```python
from build123d import *

# Parameters (mm, degrees)
SKETCH1_W           = 400
SKETCH1_H           = 300
BOSS_EXTRUDE1_DEPTH = 7.62
CUT_EXTRUDE1_DEPTH  = 7.62
CUT_EXTRUDE2_DEPTH  = 7.62


with BuildPart() as part:
    # Sketch1 → Boss-Extrude1 (new body)
    with BuildSketch(Plane(origin=(0, 0, 0), x_dir=(1, 0, 0), z_dir=(0, 1, 0))):
        with Locations((200, 150)):
            Rectangle(SKETCH1_W, SKETCH1_H)
    extrude(amount=BOSS_EXTRUDE1_DEPTH)

    # Sketch2 → Cut-Extrude1 (cut)
    with BuildSketch(Plane(origin=(0, 7.62, 0), x_dir=(1, 0, 0), z_dir=(0, 1, 0))):
        with BuildLine():
            ThreePointArc((32.1719512, 167.526), (25, 150), (32.1719512, 132.474))
            ThreePointArc((32.1719512, 132.474), (50, 89.948), (67.8280488, 132.474))
            ThreePointArc((67.8280488, 132.474), (75, 150), (67.8280488, 167.526))
            ThreePointArc((67.8280488, 167.526), (50, 210.052), (32.1719512, 167.526))
        make_face()
        with BuildLine():
            ThreePointArc((367.8280488, 167.526), (375, 150), (367.8280488, 132.474))
            ThreePointArc((367.8280488, 132.474), (350, 89.948), (332.1719512, 132.474))
            ThreePointArc((332.1719512, 132.474), (325, 150), (332.1719512, 167.526))
            ThreePointArc((332.1719512, 167.526), (350, 210.052), (367.8280488, 167.526))
        make_face()
    extrude(amount=-CUT_EXTRUDE1_DEPTH, mode=Mode.SUBTRACT)

    # Sketch3 → Cut-Extrude2 (cut)
    with BuildSketch(Plane(origin=(0, 7.62, 0), x_dir=(1, 0, 0), z_dir=(0, 1, 0))):
        with BuildLine():
            Line((180, 0), (220, 0))
            Line((220, 0), (220, 50))
            ThreePointArc((220, 50), (217.071067812, 57.071067812), (210, 60))
            Line((210, 60), (190, 60))
            ThreePointArc((190, 60), (182.928932188, 57.071067812), (180, 50))
            Line((180, 50), (180, 0))
        make_face()
    extrude(amount=-CUT_EXTRUDE2_DEPTH, mode=Mode.SUBTRACT)


solid = part.part
```
Work out the finished part from the listing and answer in its coordinate system (mm). A direction names the side the tool comes from. Give positions to 0.01 mm unless a question says otherwise; leave off trailing zeros. Write each loop counter-clockwise with the first axis right and the second up, starting at its lowest first coordinate (ties: lowest second). Pieces come first, ordered by that corner, then holes.
(1) The part is cut by section A-A on x = 50. Write down the section's boundary in (y, z), plus the area to 3 significant figures.
Final values:
outline: (0, -300) - (7.62, -300) - (7.62, -210.05) - (0, -210.05) - close; (0, -89.95) - (7.62, -89.95) - (7.62, 0) - (0, 0) - close
area: 1,370 mm2
(2) Flat-ended cylindrical pins translate along their axes: pin 1 Ø4 at (x, y) = (195.5, 2.5) entering from +Z; pin 2 Ø6 at (x, z) = (125, -146.5) entering from -Y. Find the tip coordinate at first contact, or state that the pin passes through.
Final values:
pin 1: stops at z = -60
pin 2: stops at y = 0
(3) Which of the six approach directions +Z, -Z, +X, -X, +Y, -Y give full straight-line access (tool end or side, diameter ignored) to faces 4 (the cylindrical face through (375, 4, -150)), 5 (the flat face through (197, 7.62, -152)), 6 (the cylindrical face through (217.15, 3.86, -56.99))?
Final values:
face 4: +Y, -Y
face 5: +Z, -Z, +X, -X, +Y
face 6: +Z, +Y, -Y
(4) The part is cut by section B-B on y = 5. Write down the section's boundary in (x, z), plus the area to 3 significant figures.
Final values:
outline: (0, -300) - (400, -300) - (400, 0) - (220, 0) - (220, -50) arc R10 cw to (210, -60) - (190, -60) arc R10 cw to (180, -50) - (180, 0) - (0, 0) - close; hole (32.17, -167.53) arc R25 ccw (long way) to (67.83, -167.53) arc R25 ccw to (67.83, -132.47) arc R25 ccw (long way) to (32.17, -132.47) arc R25 ccw to start; hole (332.17, -167.53) arc R25 ccw (long way) to (367.83, -167.53) arc R25 ccw to (367.83, -132.47) arc R25 ccw (long way) to (332.17, -132.47) arc R25 ccw to start
area: 107,000 mm2
(5) The part is cut by section C-C on z = -104. Write down the section's boundary in (x, y), plus the area to 3 significant figures.
Final values:
outline: (0, 0) - (27.52, 0) - (27.52, 7.62) - (0, 7.62) - close; (72.48, 0) - (327.52, 0) - (327.52, 7.62) - (72.48, 7.62) - close; (372.48, 0) - (400, 0) - (400, 7.62) - (372.48, 7.62) - close
area: 2,360 mm2
(6) The mould has two halves that part along X. Classify faces 1 (the flat face through (89, 4, 0)), 2 (the flat face through (400, 4, -148)), 3 (the cylindrical face through (350.82, 3.86, -89.96)): pulls with the +X half, pulls with the -X half, needs draft (parallel to the pull), parting line crosses it, or undercut.
Final values:
face 1: needs draft
face 2: pulls with the +X half
face 3: undercut
(7) Straight lines are drawn through the part: line 1 (X direction, y = 6.25, z = -151.5); line 2 (Z direction, x = 50, y = 6); line 3 (X direction, y = 2.5, z = -104.5). For each, find the intervals that lie inside material, in ascending order.
Final values:
line 1: x = 0 to 25.05, 74.95 to 325.05, 374.95 to 400
line 2: z = -300 to -210.05, -89.95 to 0
line 3: x = 0 to 27.29, 72.71 to 327.29, 372.71 to 400
